The listing builds one solid part. Answer for the finished solid, in the listing's coordinates (mm). A direction names the side the tool comes from. Give positions to 0.01 mm unless a question says otherwise; leave off trailing zeros. Order: outer loops, then holes, each group sorted by start corner. A loop starts at its lowest first (then second) coordinate and runs counter-clockwise, first axis right, second up. Notation, with made-up numbers: (-14, -32.75) - (17, -32.75) arc R16 cw to (17, -10.75) - close; hole circle Ø10 at (57.25, -15.5). An arc over 180 degrees is marked (long way). Answer as a JSON object with one key per item and string values. Group by question number.
Q1. For faces 5 (the face through (0.5, 0, 12)), 6 (the face through (-1.587, 0.035, 10.301)), 7 (the face through (0, 2, 9.525)), 8 (the face through (-0.5, 0, -12)), 9 (the face through (1.587, -0.035, -10.301)), determine the directions among +Z, -Z, +X, -X, +Y, -Y from which every point of the face is accessible in a straight line to the end or side of a thin tool.
Q2. Consider line 1 (Z direction, x = -0.35, y = 2) (3 decimals); line 2 (X direction, y = -1.85, z = 5); line 3 (Y direction, x = 1.35, z = -4.5). Determine where each line is inside the solid, lowest interval first.
Q3. Given pin 1 (1.5 mm diameter, centred on y = 0, z = 11.5, fed in from -X); pin 2 (2.5 mm diameter, centred on y = 0, z = 11, fed in from +X), each flat-ended and moving along its own axis, determine where each tip first touches the part or whether it passes through.
Q4. A cutting plane is placed at B-B, the plane z = -8.25. Give the vertices of the cut face in (x, y), and give its area (3 significant figures).
Q5. The mould has two halves that part along Z. Classify faces 1 (the face through (-0.5, 0, 12)), 2 (the face through (-1.74, 0.15, 11.1)), 3 (the face through (-1.655, 0.031, -12.396)), 4 (the face through (1, 0, 13.081)): released by +Z, released by -Z, zero draft, split by the parting line, or undercut.
Q6. A cutting plane is placed at C-C, the plane z = 10.75. Give the vertices of the cut face in (x, y) (1 decimal).
from build123d import *

# Parameters (mm, degrees)
F0_R           = 2.286
F1_DEPTH       = 9.525
F3_R           = 1.5875
F4_DEPTH       = 1.5748
F6_R           = 1.9875
F8_DEPTH       = 0.25
F9_R           = 1.4375
F8_FACE_R      = 1.9875
F12_DEPTH      = 2.287
F12_DEPTH_BACK = 2.287


with BuildPart() as f1:
    # F0 (on Top) → F1 (new body)
    with BuildSketch(Plane.XY):
        Circle(F0_R)
    extrude(amount=F1_DEPTH)

    # F3 (on offset) → F4 (join)
    with BuildSketch(Plane.XY.offset(9.525)):
        Circle(F3_R)
    extrude(amount=F4_DEPTH)

    # F6 (on offset) → F8 (join)
    with BuildSketch(Plane.XY.offset(11.0998)):
        Circle(F6_R)
    extrude(amount=F8_DEPTH)

    # F9 (on offset) → F10 section 0
    with BuildSketch(Plane.XY.offset(13.081)):
        Circle(F9_R)
    # F8_face (on face) → F10 section 1
    with BuildSketch(Plane.XY.offset(11.3498)):
        Circle(F8_FACE_R)
    loft()

    # F11 (on Front) → F12 (cut, two sides)
    with BuildSketch(Plane.XZ) as f12_sk:
        with BuildLine():
            Line((0.5, 13.081), (-0.5, 13.081))
            Line((-0.5, 13.081), (-0.5, 10.025))
            ThreePointArc((-0.5, 10.025), (-0.3535533906, 9.6714466094), (0, 9.525))
            ThreePointArc((0, 9.525), (0.3535533906, 9.6714466094), (0.5, 10.025))
            Line((0.5, 10.025), (0.5, 13.081))
        make_face()
    extrude(amount=-F12_DEPTH, mode=Mode.SUBTRACT)
    extrude(f12_sk.sketch, amount=F12_DEPTH_BACK, mode=Mode.SUBTRACT)

    # F13: F1 across plane


with BuildPart() as f1_1:
    add(f1.part)
    add(f1.part.mirror(Plane.XY))


solid = f1_1.part
Reply:
{
 "1": {"face 5": "+Z, +Y, -Y", "face 6": "-X", "face 7": "none", "face 8": "-Z, +Y, -Y", "face 9": "+X"},
 "2": {"line 1": "z = -9.525 to 9.525", "line 2": "x = -1.34 to 1.34", "line 3": "y = -1.84 to 1.84"},
 "3": {"pin 1": "stops at x = -1.99", "pin 2": "stops at x = 1.99"},
 "4": {"outline": "circle Ø4.57 at (0, 0)", "area": "16.4 mm^2"},
 "5": {"face 1": "zero draft", "face 2": "undercut", "face 3": "released by -Z", "face 4": "released by +Z"},
 "6": {"outline": "(-0.5, -1.5) - (-0.5, 1.5) arc R1.6 ccw to start; (0.5, -1.5) arc R1.6 ccw to (0.5, 1.5) - close"}
}
